from build123d import *
from build123d.topology import SkipClean

# Parameters (mm, degrees)
SKETCH1_W             = 26
SKETCH1_H             = 6
BOSS_EXTRUDE1_DEPTH   = 28.7
SKETCH4_R             = 1.7
CUT_EXTRUDE2_DEPTH    = 9
SKETCH8_R             = 1.7
CUT_EXTRUDE4_DEPTH    = 32.649486568
FILLET2_R             = 3
SKETCH9_R             = 22.5
CUT_EXTRUDE5_DEPTH    = 45
EXTRUDE_2_OUTLINE_W   = 50
EXTRUDE_2_OUTLINE_H   = 50
EXTRUDE_2_OUTLINE_R   = 1.5
EXTRUDE_2_OUTLINE_R_2 = 3.05
EXTRUDE_2_OUTLINE_R_3 = 1.7
EXTRUDE_2_DEPTH       = 13


# Read off the part's stored shape, not the designer's step: the extrude step
with BuildPart() as part:
    # Sketch1 → Boss-Extrude1 (new body)
    with BuildSketch(Plane.XY):
        Rectangle(SKETCH1_W, SKETCH1_H)
    extrude(amount=BOSS_EXTRUDE1_DEPTH)

    # Sketch4 → Cut-Extrude2 (cut)
    with BuildSketch(Plane(origin=(0, 0, 0), x_dir=(-1, 0, 0), z_dir=(0, 0, -1))):
        with Locations((10, 0)):
            Circle(SKETCH4_R)
    extrude(amount=-CUT_EXTRUDE2_DEPTH, mode=Mode.SUBTRACT)

    # Sketch8 → Cut-Extrude4 (cut, through all)
    with BuildSketch(Plane.XY.offset(28.7)):
        with Locations(Location((-10, 0, 0), (0, 0, 180))):
            Circle(SKETCH8_R)
        with Locations((10, 0)):
            Circle(SKETCH8_R)
    extrude(amount=-CUT_EXTRUDE4_DEPTH, mode=Mode.SUBTRACT)

    # Fillet2
    fillet2_edges = [part.edges().sort_by_distance(p)[0] for p in [
        (13, -3, 14.35),
        (-13, -3, 14.35),
    ]]
    fillet(fillet2_edges, radius=FILLET2_R)

    # Sketch9 → Cut-Extrude5 (cut)
    with BuildSketch(Plane(origin=(0, 0, 0), x_dir=(-1, 0, 0), z_dir=(0, 0, -1))):
        with Locations((0, -23)):
            Circle(SKETCH9_R)
    extrude(amount=-CUT_EXTRUDE5_DEPTH, mode=Mode.SUBTRACT)

    # Extrude 2 outline → Extrude 2 (add)
    with SkipClean():  # the faces are left unmerged after this step: merging them gives an invalid solid
        with BuildSketch(Plane.XY.offset(28.7)):
            with Locations((0, -21.940687277)):
                Rectangle(EXTRUDE_2_OUTLINE_W, EXTRUDE_2_OUTLINE_H)
            with Locations((-11.95, -35.590687277)):
                Circle(EXTRUDE_2_OUTLINE_R, mode=Mode.SUBTRACT)
            with Locations((11.95, -35.590687277)):
                Circle(EXTRUDE_2_OUTLINE_R, mode=Mode.SUBTRACT)
            with Locations((0, -23.640687277)):
                Circle(EXTRUDE_2_OUTLINE_R_2, mode=Mode.SUBTRACT)
            with Locations((-11.95, -11.690687277)):
                Circle(EXTRUDE_2_OUTLINE_R, mode=Mode.SUBTRACT)
            with Locations((-10, 0)):
                Circle(EXTRUDE_2_OUTLINE_R_3, mode=Mode.SUBTRACT)
            with Locations((11.95, -11.690687277)):
                Circle(EXTRUDE_2_OUTLINE_R, mode=Mode.SUBTRACT)
            with Locations((10, 0)):
                Circle(EXTRUDE_2_OUTLINE_R_3, mode=Mode.SUBTRACT)
        extrude(amount=EXTRUDE_2_DEPTH)
    add(part.part.scale(1), mode=Mode.REPLACE)  # the faces are merged on a copy


solid = part.part
Geometry check sheet. Reference: the model listing, model coordinates, mm. A direction names the side the tool comes from. Give positions to 0.01 mm unless a question says otherwise; leave off trailing zeros. Loops run counter-clockwise (first coordinate to the right, second up) from the corner with the lowest first, then second, coordinate; pieces in that order, holes last. Notation, with made-up numbers: M 82,-27 L 131,-27 A15 ccw 131,-23 Z; hole C 24.25,50 d8. An arc over 180 degrees is marked long. Answer as a JSON object with one key per item and string values. Group by question number.
Item 1: Sectioned sample at D-D on x = -6. Record the boundary of the cut face in (y, z), plus the area to 3 significant figures.
Item 2: Mould release check, pull along X, two halves, no side actions. Record for faces 1 (the cylindrical face through (-10.52, -11.24, 35.11)), 2 (the flat face through (-13, 1, 14)), 3 (the cylindrical face through (-0.397, -20.617, 35.109)), 4 (the flat face through (0, -46.941, 35)): pulls with the +X half, pulls with the -X half, needs draft (parallel to the pull), parting line crosses it, or undercut.
Item 3: Material ranges on L1, parallel to Y at x = -11.95, z = 33.75; L2, parallel to Y at x = 10, z = 36.5; L3, parallel to Y at x = -11, z = 38, recorded low to high.
Item 4: Access from +Z, -Z, +X, -X, +Y, -Y to the whole of each face (thin tool, end or side, straight path). Record for faces 5 (the flat face through (13, 1, 14)), 6 (the cylindrical face through (-12.24, -1.996, 14.551)), 7 (the flat face through (0, 3, 14)), 8 (the cylindrical face through (12.24, -1.996, 14.551)).
Item 5: Sectioned sample at A-A on x = 0. Record the boundary of the cut face in (y, z), plus the area to 3 significant figures.
Item 6: Gauge pin test, flat ends, axial feed: pin 1 (6 mm diameter, centred on x = -2, y = -6, fed in from -Z); pin 2 (2.5 mm diameter, centred on y = 2, z = 8.5, fed in from +X); pin 3 (4.5 mm diameter, centred on x = -10, y = 0, fed in from -Z); pin 4 (2.5 mm diameter, centred on x = -11.95, y = -35.59, fed in from +Z). Record the tip position at first contact, or that the pin passes through.
Item 7: Sectioned sample at B-B on y = -12.5. Record the boundary of the cut face in (x, z), plus the area to 3 significant figures.
Item 8: Sectioned sample at C-C on z = 16. Record the boundary of the cut face in (x, y).
Findings below:
{
 "1": {"outline": "M -46.94,28.7 L -1.31,28.7 L -1.31,0 L 3,0 L 3,28.7 L 3.06,28.7 L 3.06,41.7 L -46.94,41.7 Z", "area": "774 mm2"},
 "2": {"face 1": "undercut", "face 2": "pulls with the -X half", "face 3": "undercut", "face 4": "needs draft"},
 "3": {"L1": "-46.94 to -37.09, -34.09 to -13.19, -10.19 to 3.06", "L2": "-46.94 to -1.7, 1.7 to 3.06", "L3": "-46.94 to -36.75, -34.43 to -12.85, -10.53 to -1.37, 1.37 to 3.06"},
 "4": {"face 5": "-Z, +X, +Y, -Y", "face 6": "-Z, -X, -Y", "face 7": "-Z, +X, -X, +Y", "face 8": "-Z, +X, -Y"},
 "5": {"outline": "M -46.94,28.7 L -26.69,28.7 L -26.69,41.7 L -46.94,41.7 Z; M -20.59,28.7 L -0.5,28.7 L -0.5,0 L 3,0 L 3,28.7 L 3.06,28.7 L 3.06,41.7 L -20.59,41.7 Z", "area": "671 mm2"},
 "6": {"pin 1": "z = 28.7", "pin 2": "x = 13", "pin 3": "z = 0", "pin 4": "through"},
 "7": {"outline": "M -25,28.7 L -13.21,28.7 L -13.21,41.7 L -25,41.7 Z; M -10.69,28.7 L 10.69,28.7 L 10.69,41.7 L -10.69,41.7 Z; M 13.21,28.7 L 25,28.7 L 25,41.7 L 13.21,41.7 Z", "area": "584 mm2"},
 "8": {"outline": "M -13,0 A3 ccw -10.28,-2.99 A22.5 cw 10.28,-2.99 A3 ccw 13,0 L 13,3 L -13,3 Z; hole C -10,0 d3.4; hole C 10,0 d3.4"}
}
